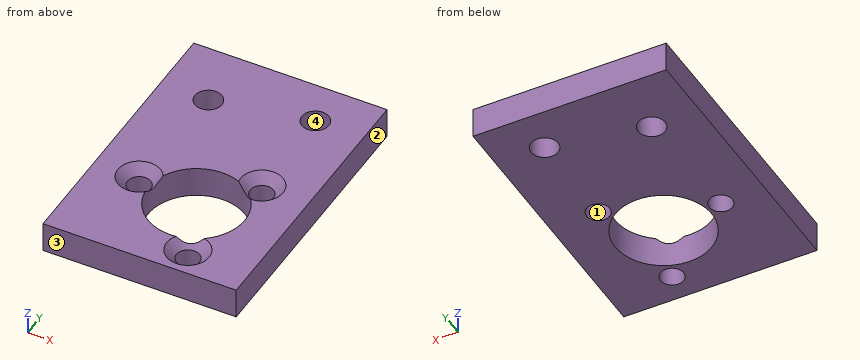
from build123d import *

# Parameters (mm, degrees)
SKETCH1_W                                       = 20
SKETCH1_H                                       = 29.11
SKETCH1_R                                       = 1.4
SKETCH1_R_2                                     = 1.2
SKETCH1_R_3                                     = 5
BOSS_EXTRUDE2_DEPTH                             = 3.18
CSK_FOR_M2_FLAT_HEAD_MACHINE_SCREW1_D           = 2.4
CSK_FOR_M2_FLAT_HEAD_MACHINE_SCREW1_DEPTH       = 3.508967257
CSK_FOR_M2_FLAT_HEAD_MACHINE_SCREW1_CSINK_D     = 4.4
CSK_FOR_M2_FLAT_HEAD_MACHINE_SCREW1_CSINK_ANGLE = 90
CSK_FOR_M2_FLAT_HEAD_MACHINE_SCREW1_TIP         = 0.721032743


with BuildPart() as part:
    # Sketch1 → Boss-Extrude2 (new body)
    with BuildSketch(Plane.XY):
        with Locations((10, 14.555)):
            Rectangle(SKETCH1_W, SKETCH1_H)
        with Locations((5, 22.61)):
            Circle(SKETCH1_R, mode=Mode.SUBTRACT)
        with Locations((15, 24.61)):
            Circle(SKETCH1_R, mode=Mode.SUBTRACT)
        with Locations((15.03, 14.21)):
            Circle(SKETCH1_R_2, mode=Mode.SUBTRACT)
        with Locations((4.57, 10.04)):
            Circle(SKETCH1_R_2, mode=Mode.SUBTRACT)
        with Locations((13.41, 2.96)):
            Circle(SKETCH1_R_2, mode=Mode.SUBTRACT)
        with Locations((11, 9.11)):
            Circle(SKETCH1_R_3, mode=Mode.SUBTRACT)
    extrude(amount=-BOSS_EXTRUDE2_DEPTH)

    # CSK for M2 Flat Head Machine Screw1
    with Locations(Plane.XY):
        with Locations((4.57, 10.04), (15.03, 14.21), (13.41, 2.96)):
            CounterSinkHole(CSK_FOR_M2_FLAT_HEAD_MACHINE_SCREW1_D / 2, CSK_FOR_M2_FLAT_HEAD_MACHINE_SCREW1_CSINK_D / 2, depth=CSK_FOR_M2_FLAT_HEAD_MACHINE_SCREW1_DEPTH, counter_sink_angle=CSK_FOR_M2_FLAT_HEAD_MACHINE_SCREW1_CSINK_ANGLE)
            with Locations((0, 0, -(CSK_FOR_M2_FLAT_HEAD_MACHINE_SCREW1_DEPTH + CSK_FOR_M2_FLAT_HEAD_MACHINE_SCREW1_TIP / 2))):  # 118° drill point
                Cone(0, CSK_FOR_M2_FLAT_HEAD_MACHINE_SCREW1_D / 2, CSK_FOR_M2_FLAT_HEAD_MACHINE_SCREW1_TIP, mode=Mode.SUBTRACT)


solid = part.part
The model under review builds one solid part; all positions refer to its coordinate system, in mm. Face numbers are marked on the shaded views. Round coordinates to 2 decimals unless told otherwise and drop trailing zeros. Loops run counter-clockwise (first coordinate to the right, second up) from the corner with the lowest first, then second, coordinate; pieces in that order, holes last. Notation, with made-up numbers: M 66.5,-15 L 113.5,-15 A11 cw 113.5,0 Z; hole C 28,-16.5 d3. An arc over 180 degrees is marked long. Answer as a JSON object with one key per item and string values.
Item 1: Clearance check with flat-ended pins moving along their axes: P1, Ø3, axis at x = 13.41, y = 2.96, coming from the +Z side; P2, Ø4, axis at x = 4.57, y = 10.04, coming from the +Z side. State where each tip first meets the part, or that it passes through.
Check sheet entries:
{"P1": "z = -0.7", "P2": "z = -0.2"}
Item 2: We need section A-A, the plane y = 2.96. State the section outline as (x, z) points, and give its area (3 significant figures).
Check sheet entries:
{"outline": "M 0,-3.18 L 12.21,-3.18 L 12.21,-1 L 11.21,0 L 0,0 Z; M 14.61,-3.18 L 20,-3.18 L 20,0 L 15.61,0 L 14.61,-1 Z", "area": "55.0 mm2"}
Item 3: We need section C-C, the plane x = 10.25. State the section outline as (y, z) points.
Check sheet entries:
{"outline": "M 0,-3.18 L 4.17,-3.18 L 4.17,0 L 0,0 Z; M 14.05,-3.18 L 29.11,-3.18 L 29.11,0 L 14.05,0 Z"}
Item 4: We need section B-B, the plane z = -1.7. State the section outline as (x, y) points.
Check sheet entries:
{"outline": "M 0,0 L 20,0 L 20,29.11 L 0,29.11 Z; hole C 4.57,10.04 d2.4; hole C 5,22.61 d2.8; hole C 11,9.11 d10; hole C 13.41,2.96 d2.4; hole C 15,24.61 d2.8; hole C 15.03,14.21 d2.4"}
Item 5: We need section D-D, the plane y = 10.04. State the section outline as (x, z) points.
Check sheet entries:
{"outline": "M 0,-3.18 L 3.37,-3.18 L 3.37,-1 L 2.37,0 L 0,0 Z; M 5.77,-3.18 L 6.09,-3.18 L 6.09,-0.68 L 5.77,-1 Z; M 15.91,-3.18 L 20,-3.18 L 20,0 L 15.91,0 Z"}
Item 6: For line 1 along X through (y, z) = (11, -2.9); line 2 along X through (y, z) = (11.75, -0.25); line 3 along Y through (x, z) = (10.75, -0.9), list the stretches that pass through material, from the lowest coordinate up.
Check sheet entries:
{"line 1": "0 to 3.85, 5.29 to 6.37, 15.63 to 20", "line 2": "0 to 3.63, 5.51 to 6.75, 15.25 to 20", "line 3": "0 to 4.12, 14.1 to 29.11"}
Item 7: The part is to be moulded in two halves that separate along Y. For the marked faces 1, 2, 3 and 4, say which applies: +Y half, -Y half, draft (parallel to the pull), parting line (faces both ways), or undercut.
Check sheet entries:
{"face 1": "undercut", "face 2": "draft", "face 3": "-Y half", "face 4": "undercut"}
